Can you work these out from the model? Positions are in its coordinate system, mm. Face numbers are marked on the shaded views. Round coordinates to 2 decimals unless told otherwise and drop trailing zeros. Loops run counter-clockwise (first coordinate to the right, second up) from the corner with the lowest first, then second, coordinate; pieces in that order, holes last. Notation, with made-up numbers: M 85.5,65 L 114.5,65 A12 ccw 114.5,75 Z; hole C 3,66 d4. An arc over 180 degrees is marked long. Return JSON: item names as keys, results as strings.
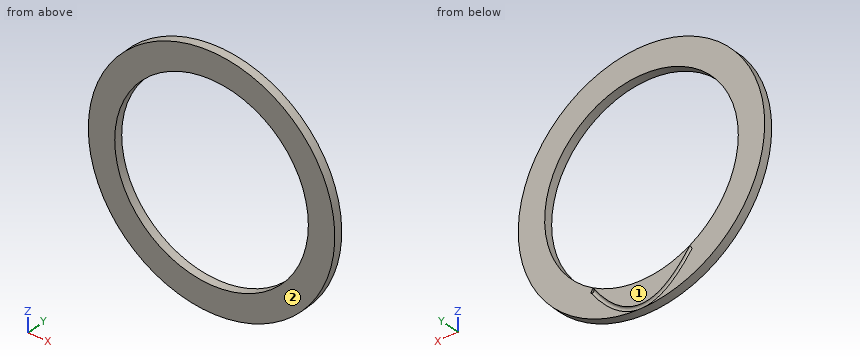
Autodesk Inventor part; units mm, degrees
ref_plane "Work Plane3" through (0, 0, 0) normal (0.8660254, 0, 0.5) x (0.5, 0, -0.8660254)
ref_plane "Work Plane4" through (0, 0, 0) normal (-1, 0, 0) x (0, 0, -1)
ref_plane "Work Plane5" through (0, 0, 0) normal (0.8660254, 0, -0.5) x (-0.5, 0, -0.8660254)
sketch "Sketch1" plane through (0, 0, 0) normal (0, 1, 0) x (-1, 0, 0)
  circle A0 centre (0, 0) radius 139.7
  circle A1 centre (0, 0) radius 177.8
  dimension "innerDiameter" = 279.4
  dimension "outerDiameter" = 355.6
extrude "Extrusion1" add sketch "Sketch1" against normal blind 12.7
sketch "Sketch5" plane through (0, 0, 0) normal (0, 1, 0) x (1, 0, 0)
  line L0 (0, 0) -> (-88.9, 153.9793) construction
  circle A0 centre (0, 0) radius 177.8 construction
  line L1 (0, 0) -> (88.9, 153.9793) construction
  line L2 (0, 0) -> (0, 177.8) construction
  circle A1 centre (0, 0) radius 142.875 construction
  circle A2 centre (0, 0) radius 174.625 construction
  point P0 (71.4375, 123.7334)
  point P1 (0, 174.625)
  point P2 (-71.4375, 123.7334)
  dimension "camOuterDiameter" = 349.25
  dimension "arcForCam" = 30
  dimension "d12" = 30
  dimension "camInnerDiameter" = 285.75
ref_plane "Work Plane3" through (0, 0, 0) normal (0.8660254, 0, 0.5) x (0.5, 0, -0.8660254)
ref_plane "Work Plane4" through (0, 0, 0) normal (-1, 0, 0) x (0, 0, -1)
ref_plane "Work Plane5" through (0, 0, 0) normal (0.8660254, 0, -0.5) x (-0.5, 0, -0.8660254)
sketch "Sketch10" plane through (0, 0, 0) normal (0.8660254, 0, 0.5) x (0.5, 0, -0.8660254)
  line L0 (-177.8, 0) -> (177.8, 0)
  circle A0 centre (142.875, 0) radius 3.175
  point P0 (0, 0)
  dimension "camDiameter" = 6.35
  dimension "d30" = 142.875
sketch "Sketch12" plane through (0, 0, 0) normal (-1, 0, 0) x (0, 0, -1)
  circle A0 centre (174.625, 0) radius 3.175
  point P0 (0, 0)
  dimension "d31" = 174.625
  dimension "d32" = 6.35
sketch "Sketch13" plane through (0, 0, 0) normal (0.8660254, 0, -0.5) x (-0.5, 0, -0.8660254)
  circle A0 centre (142.875, 0) radius 3.175
  point P0 (0, 0)
  dimension "d33" = 6.35
  dimension "d34" = 142.875
loft "Loft2" cut profiles "Sketch10", "Sketch12", "Sketch13"
equation "\"d12\" = arcForCam"
equation "\"d32\" = camDiameter"
equation "\"d33\" = camDiameter"
properties part number "NewCam02"
Q1. I'm going to push flat-ended pins straight in: pin 1 Ø6 at (x, y) = (-30, -8) entering from +Z; pin 2 Ø1 at (y, z) = (-7.5, -104) entering from -X; pin 3 Ø1 at (y, z) = (-4, 58) entering from -X. Where does each tip first touch, or does it pass through?
Results:
{"pin 1": "stops at z = 175.74", "pin 2": "stops at x = -144.57", "pin 3": "stops at x = -168.25"}
Q2. Suppose I cut it at B-B, the plane x = 118.5. Please give me the cut outline in (y, z).
Results:
{"outline": "M -12.7,-132.55 L 0,-132.55 L 0,-73.99 L -12.7,-73.99 Z; M -12.7,73.99 L 0,73.99 L 0,132.55 L -12.7,132.55 Z"}
Q3. Suppose I cut it at A-A, the plane z = 0. Please give me the cut outline in (x, y), plus the area to 3 significant figures.
Results:
{"outline": "M -177.8,-12.7 L -139.7,-12.7 L -139.7,0 L -177.8,0 Z; M 139.7,-12.7 L 177.8,-12.7 L 177.8,0 L 139.7,0 Z", "area": "968 mm2"}
Q4. Thinking about a two-plate mould opening in Y: for the marked faces 1 and 2, which applies, pulls with the +Y half, pulls with the -Y half, needs draft (parallel to the pull), parting line crosses it, or undercut?
Results:
{"face 1": "pulls with the +Y half", "face 2": "pulls with the -Y half"}
Q5. Suppose I cut it at C-C, the plane y = -9. Please give me the cut outline in (x, z).
Results:
{"outline": "C 0,0 d355.6; hole C 0,0 d279.4"}
Q6. If I drill on line 1 along X through (y, z) = (-4.5, 0); line 2 along X through (y, z) = (-7, -47.5), over which ranges is the centre line in solid material (lowest first)?
Results:
{"line 1": "x = -177.8 to -139.7, 139.7 to 177.8", "line 2": "x = -171.34 to -131.38, 131.38 to 171.34"}
